Source: CAD feature listing. Evaluate the final solid. Frame: model axes, mm. Face numbers are marked on the shaded views. Give positions to 0.01 mm unless a question says otherwise; leave off trailing zeros. Write each question's results on one line, items separated by ' | '. Start each with the question number.
Item 1: Line query: line 1 along Z through (x, y) = (4.5, 3); line 2 along Y through (x, z) = (-2, 1.1); line 3 along Z through (x, y) = (4.5, -22.5). Output: solid intervals per line, ascending.
Item 2: Contact query for flat-ended pins moving along their axis: pin 1 Ø1 at (x, y) = (5, 18) entering from +Z; pin 2 Ø12 at (x, y) = (-10, -18.5) entering from -Z; pin 3 Ø12 at (x, y) = (0, 0) entering from +Z. Output: stop coordinate, or through.
Item 3: Mould query, pull axis Y, two halves, no side actions, for the marked faces 1, 2 and 3. Classes: released by +Y, released by -Y, zero draft, split by the parting line, or undercut.
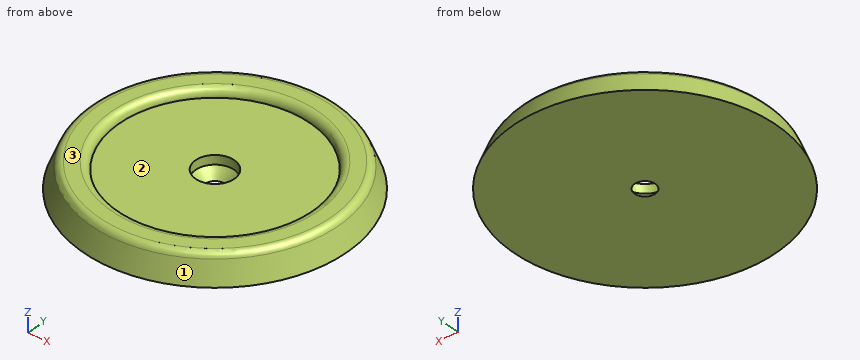
```python
from build123d import *

# Parameters (mm, degrees)
F0_R        = 18.5
F0_R_2      = 2
F1_DEPTH    = 3.5
F2_R        = 3.75
F3_DEPTH    = 0.5
F4_S5_R     = 3.75
F4_T6_DEPTH = 9
F8_R        = 1.49999


# Not quite as in the source:
# - a fillet or chamfer that OpenCascade refuses, or shapes differently, is made with other operations: its cross-section is extruded or revolved along the edge and cut away or added
# - a fillet or chamfer is up to 0.001 mm smaller than in the source, because OpenCascade refuses the exact size


with BuildPart() as f1:
    # F0 (on Top) → F1 (new body)
    with BuildSketch(Plane.XY):
        Circle(F0_R)
        Circle(F0_R_2, mode=Mode.SUBTRACT)
    extrude(amount=F1_DEPTH)

    # F2 (on face) → F3 (cut)
    with BuildSketch(Plane.XY.offset(3.5)):
        Circle(F2_R)
    extrude(amount=-F3_DEPTH, mode=Mode.SUBTRACT)

    # F4: chamfer of 3 on 1 edges, made by hand


with BuildPart() as f4_tool2:
    # F4_s3 → F4_t4 (revolve)
    with BuildSketch(Plane.XZ):
        Polygon((2, 0), (5, 3), (2, 3), align=None)
    revolve(axis=Axis((0, 0, 3), (0, 0, -1)))

    # F4_s5 → F4_t6 (intersect, symmetric)
    with BuildSketch(Plane.XY.offset(1.5)):
        Circle(F4_S5_R)
    extrude(amount=F4_T6_DEPTH, both=True, mode=Mode.INTERSECT)


with BuildPart() as f1_1:
    add(f1.part)

    # F4_t1: cut F4_tool2
    add(f4_tool2.part, mode=Mode.SUBTRACT)

    # F6 (on Right) → F7 (revolve)
    with BuildSketch(Plane.YZ):
        Polygon((-25.5, 0), (-18.5, 0), (-18.5, 3.5), (-18.5, 5), (-23.5, 5), align=None)
    revolve(axis=Axis((0, 0, 7.0907436311), (0, 0, 1)))

    # F8 (radius 1.5 in the source; OpenCascade refuses exactly that, so slightly less here)
    f8_edges = [f1_1.edges().sort_by_distance(p)[0] for p in [
        (0, 23.5, 5),
        (0, 18.5, 5),
    ]]
    fillet(f8_edges, radius=F8_R)


solid = f1_1.part
```
Evaluation:
1) line 1: z = 0 to 3.5 | line 2: y = -24.98 to -2.37, 2.37 to 24.98 | line 3: z = 0 to 4.93
2) pin 1: stops at z = 4.76 | pin 2: stops at z = 0 | pin 3: stops at z = 3.5
3) face 1: split by the parting line | face 2: undercut | face 3: zero draft
